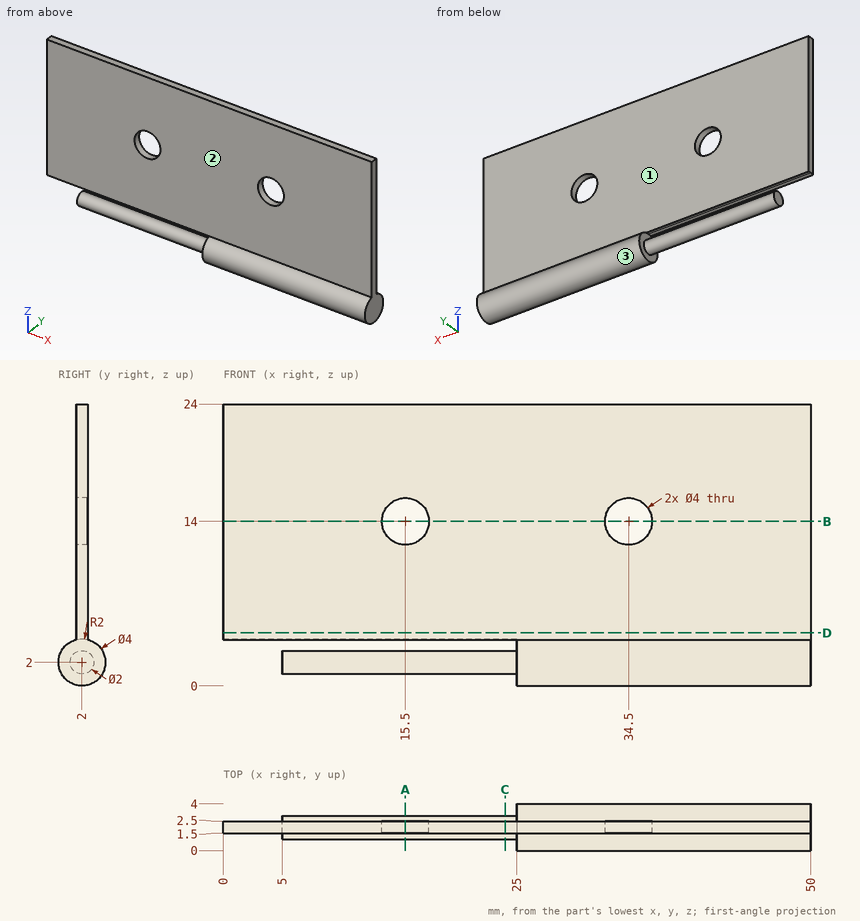
Can you work these out from the drawing? Everything is in mm from the part's minimum corner. A direction names the side the tool comes from. Round coordinates to 2 decimals unless told otherwise and drop trailing zeros. Write each loop counter-clockwise with the first axis right and the second up, starting at its lowest first coordinate (ties: lowest second). Pieces come first, ordered by that corner, then holes. Notation, with made-up numbers: (61.5, 3.5) - (110.5, 3.5) arc R19 cw to (110.5, 14.5) - close; hole circle Ø2 at (60.5, 11). An arc over 180 degrees is marked (long way). Write each question's results on one line, items separated by ' | '. Start each with the question number.
1) Suppose I cut it at A-A (x = 15.5). List the corners of the cut face in (y, z) for me.
2) Suppose I cut it at D-D (z = 4.5). List the corners of the cut face in (x, y) for me, and give its area (3 significant figures).
3) Please list where these lines run through material, in increasing order: line 1 (X direction, y = 1.7, z = 14); line 2 (Z direction, x = 15.5, y = 1.85); line 3 (X direction, y = 1.7, z = 15.75).
4) For pin 1 Ø12 at (x, z) = (35.5, 7.5) entering from -Y; pin 2 Ø5 at (x, z) = (20, 9.5) entering from -Y; pin 3 Ø3.5 at (x, z) = (15.5, 14) entering from -Y; pin 4 Ø10 at (x, z) = (10.5, 14.5) entering from +Y, each with a flat end and sliding along its axis, tell me the tip position at first contact or that it passes through.
5) Suppose I cut it at C-C (x = 24). List the corners of the cut face in (y, z) for me, and give its area (3 significant figures).
6) Suppose I cut it at B-B (z = 14). List the corners of the cut face in (x, y) for me, and give its area (3 significant figures).
7) Which directions (+Z, -Z, +X, -X, +Y, -Y) give clear straight access to the entire face, cutting with the end or side of a thin tool? Please do the marked faces 1, 2 and 3.
Here are the results:
1) outline: circle Ø2 at (2, 2); (1.5, 3.94) arc R2 cw to (2.5, 3.94) - (2.5, 12) - (1.5, 12) - close; (1.5, 16) - (2.5, 16) - (2.5, 24) - (1.5, 24) - close
2) outline: (0, 1.5) - (50, 1.5) - (50, 2.5) - (0, 2.5) - close | area: 50.0 mm2
3) line 1: x = 0 to 13.5, 17.5 to 32.5, 36.5 to 50 | line 2: z = 1.01 to 2.99, 3.99 to 12, 16 to 24 | line 3: x = 0 to 14.53, 16.47 to 33.53, 35.47 to 50
4) pin 1: stops at y = 0 | pin 2: stops at y = 1.5 | pin 3: passes through | pin 4: stops at y = 2.5
5) outline: circle Ø2 at (2, 2); (1.5, 3.94) arc R2 cw to (2.5, 3.94) - (2.5, 24) - (1.5, 24) - close | area: 23.2 mm2
6) outline: (0, 1.5) - (13.5, 1.5) - (13.5, 2.5) - (0, 2.5) - close; (17.5, 1.5) - (32.5, 1.5) - (32.5, 2.5) - (17.5, 2.5) - close; (36.5, 1.5) - (50, 1.5) - (50, 2.5) - (36.5, 2.5) - close | area: 42.0 mm2
7) face 1: +Z, +X, -X, +Y | face 2: +Z, +X, -X, -Y | face 3: +X, -X
